Autodesk Inventor part; units mm, degrees
ref_plane "YZ Plane" through (0, 0, 0) normal (1, 0, 0) x (0, 1, 0)
ref_plane "XZ Plane" through (0, 0, 0) normal (0, 1, 0) x (-1, 0, 0)
ref_plane "XY Plane" through (0, 0, 0) normal (0, 0, 1) x (1, 0, 0)
sketch "Sketch1" plane through (0, 0, 0) normal (0, 0, 1) x (1, 0, 0)
  line L0 (0, 0) -> (0, 24.13)
  line L1 (0, 24.13) -> (24.13, 24.13)
  line L2 (24.13, 24.13) -> (24.13, 0)
  line L3 (24.13, 0) -> (0, 0)
  line L4 (0, 0) -> (0, 1.7526)
  line L5 (9.144, 1.7526) -> (14.986, 1.7526)
  line L6 (9.144, 1.7526) -> (9.271, 1.7526)
  line L7 (9.271, 1.7526) -> (14.859, 1.7526)
  line L8 (0, 0) -> (0, 7.62)
  line L9 (24.13, 0) -> (24.13, 7.62)
  line L10 (14.859, 7.62) -> (19.685, 7.62)
  line L11 (19.685, 7.62) -> (19.685, 12.319)
  line L12 (19.685, 12.319) -> (14.859, 12.319)
  line L13 (9.271, 7.62) -> (4.445, 7.62)
  line L14 (4.445, 7.62) -> (4.445, 12.319)
  line L15 (4.445, 12.319) -> (9.271, 12.319)
  line L16 (9.271, 7.62) -> (9.271, 1.7526)
  line L17 (14.859, 1.7526) -> (14.859, 7.62)
  line L18 (14.859, 12.319) -> (14.859, 15.748)
  line L19 (9.271, 12.319) -> (9.271, 15.748)
  line L20 (19.812, 15.748) -> (19.812, 19.685)
  line L21 (14.859, 15.748) -> (19.812, 15.748)
  line L22 (19.812, 19.685) -> (4.445, 19.685)
  line L23 (4.445, 19.685) -> (4.445, 15.748)
  line L24 (4.445, 15.748) -> (9.271, 15.748)
  dimension "d0" = 24.13
  dimension "d1" = 24.13
  dimension "d2" = 1.7526
  dimension "d3" = 9.144
  dimension "d5" = 0.127
  dimension "d6" = 5.588
  dimension "d7" = 7.62
  dimension "d8" = 7.62
  dimension "d9" = 4.826
  dimension "d10" = 4.699
  dimension "d11" = 4.826
  dimension "d12" = 4.699
  dimension "d13" = 5.8674
  dimension "d14" = 5.8674
  dimension "d15" = 3.429
  dimension "d16" = 3.429
  dimension "d18" = 3.937
sketch "Sketch2" plane through (0, 0, 0) normal (0, 0, 1) x (1, 0, 0)
  point P0 (0, 0)
extrude "Extrusion1" add sketch "Sketch1" along normal blind 152.4
chamfer "Chamfer1" distance 6.35 angle 45 4 edges at (0, 24.13, 76.2) (24.13, 24.13, 76.2) (24.13, 0, 76.2) (0, 0, 76.2)
sketch "Sketch3" plane through (6.35, 0, 0) normal (0, -1, 0) x (1, 0, 0)
  line L0 (17.78, 0) -> (17.78, 152.4)
  line L1 (17.78, 152.4) -> (17.78, 144.78)
  line L2 (17.78, 144.78) -> (-6.35, 144.78)
  line L3 (2.921, 0) -> (2.921, 152.4)
  line L4 (-6.35, 144.78) -> (-6.35, 137.16)
  line L5 (-6.35, 152.4) -> (-6.35, 0)
  line L6 (-6.35, 137.16) -> (17.78, 137.16)
  line L7 (17.78, 137.16) -> (17.78, 144.78)
  dimension "d24" = 7.62
  dimension "d25" = 7.62
extrude "Extrusion2" cut sketch "Sketch3" against normal blind 17.399
sketch "Sketch4" plane through (6.35, 0, 0) normal (0, -1, 0) x (1, 0, 0)
  line L0 (17.78, 144.78) -> (17.78, 137.16)
  line L1 (17.78, 137.16) -> (-6.35, 137.16)
  line L2 (-6.35, 137.16) -> (-6.35, 133.604)
  line L3 (-6.35, 133.604) -> (17.78, 133.604)
  line L4 (17.78, 133.604) -> (17.78, 137.16)
  point P0 (-6.35, 0)
  dimension "d28" = 3.556
extrude "Extrusion3" add sketch "Sketch4" against normal blind 1.7526
sketch "Sketch5" plane through (0, 6.35, 137.16) normal (-0.7071, -0.7071, 0) x (-0.7071, 0.7071, 0)
  point P0 (-4.4901, 137.16)
sketch "Sketch6" plane through (6.35, 0, 0) normal (0, -1, 0) x (1, 0, 0)
  point P0 (-6.35, 0)
sketch "Sketch7" plane through (6.35, 0, 0) normal (0, -1, 0) x (1, 0, 0)
  line L0 (17.78, 137.16) -> (13.1826, 137.16)
  line L1 (-6.35, 137.16) -> (-6.35, 0)
  line L2 (17.78, 137.16) -> (-6.35, 137.16)
  line L3 (-6.35, 137.16) -> (-6.35, 133.604)
  line L4 (-6.35, 133.604) -> (17.78, 133.604)
  line L5 (17.78, 133.604) -> (17.78, 137.16)
  dimension "d31" = 3.556
extrude "Extrusion4" add sketch "Sketch7" along normal blind 3.81
chamfer "Chamfer2" distance 2.54 angle 45 1 edges at (12.065, -3.81, 133.604)
sketch "Sketch8" plane through (24.13, 1.7526, 137.16) normal (1, 0, 0) x (0, 0, -1)
  point P0 (137.16, -1.7526)
sketch "Sketch9" plane through (6.35, 1.7526, 0) normal (0, 1, 0) x (1, 0, 0)
  line L0 (17.78, -137.16) -> (17.78, -133.604)
  line L1 (13.1826, -137.16) -> (17.78, -137.16)
  line L2 (17.78, -137.16) -> (13.1826, -137.16)
  line L3 (13.1826, -137.16) -> (13.1826, -133.604)
  line L4 (13.1826, -133.604) -> (17.78, -133.604)
  line L5 (17.78, -133.604) -> (17.78, -137.16)
  point P0 (-6.35, 0)
extrude "Extrusion5" add sketch "Sketch9" along normal blind 5.08
sketch "Sketch10" plane through (6.35, 1.7526, 0) normal (0, 1, 0) x (1, 0, 0)
  point P0 (-6.35, 0)
sketch "Sketch11" plane through (0, 1.7526, 133.604) normal (-1, 0, 0) x (0, 0, 1)
  point P0 (-133.604, -1.7526)
sketch "Sketch12" plane through (0, 1.7526, 133.604) normal (-1, 0, 0) x (0, 0, 1)
  point P0 (-133.604, -1.7526)
sketch "Sketch13" plane through (6.35, 1.7526, 0) normal (0, 1, 0) x (1, 0, 0)
  line L0 (-1.7526, -133.604) -> (-1.7526, -137.16)
  line L1 (-6.35, -133.604) -> (17.78, -133.604)
  line L2 (-1.7526, -137.16) -> (-1.7526, -133.604)
  line L3 (-1.7526, -133.604) -> (-6.35, -133.604)
  line L4 (-6.35, -133.604) -> (-6.35, -137.16)
  line L5 (-6.35, -137.16) -> (-1.7526, -137.16)
  point P0 (-6.35, 0)
extrude "Extrusion6" add sketch "Sketch13" along normal blind 5.08
properties part number "RIPnewslideholder"
Geometry check sheet. Reference: the model listing, model coordinates, mm. A direction names the side the tool comes from. Give positions to 0.01 mm unless a question says otherwise; leave off trailing zeros. Write each loop counter-clockwise with the first axis right and the second up, starting at its lowest first coordinate (ties: lowest second). Pieces come first, ordered by that corner, then holes.
1) Access from +Z, -Z, +X, -X, +Y, -Y to the whole of each face (thin tool, end or side, straight path). Record for faces 4 (the flat face through (22, 17.399, 141)), 5 (the flat face through (19.685, 10, 149)), 6 (the flat face through (3.22, 21, 75.13)).
2) Material ranges on L1, parallel to Y at x = 8.5, z = 24.5 (3 decimals); L2, parallel to Z at x = 9, y = 7.5; L3, parallel to X at y = 17.5, z = 89 (3 decimals), recorded low to high.
3) Release check for a two-part mould opening along Z. For faces 1 (the flat face through (2, 17.399, 141)), 2 (the flat face through (17, 15.748, 68)), 3 (the flat face through (9, 15, 0)) record: pulls with the +Z half, pulls with the -Z half, needs draft (parallel to the pull), parting line crosses it, or undercut.
4) Section check B-B, the plane x = 21.5. Record the boundary of the cut face in (y, z), and give its area (3 significant figures).
5) Section check A-A, the plane x = 11.5. Record the boundary of the cut face in (y, z) (3 decimals).
6) Gauge pin test, flat ends, axial feed: pin 1 (6 mm diameter, centred on y = 21.5, z = 46, fed in from +X); pin 2 (1 mm diameter, centred on y = 1.5, z = 119, fed in from -X); pin 3 (5 mm diameter, centred on x = 21, z = 130, fed in from +Y). Record the tip position at first contact, or that the pin passes through.
Computed:
1. face 4: +X, -X, -Y
1. face 5: +Z, -Z
1. face 6: +Z, -Z, -X, +Y
2. L1: y = 0 to 7.62, 12.319 to 15.748, 19.685 to 24.13
2. L2: z = 0 to 137.16, 144.78 to 152.4
2. L3: x = 0 to 4.445, 19.812 to 24.13
3. face 1: undercut
3. face 2: needs draft
3. face 3: pulls with the -Z half
4. outline: (-3.81, 136.14) - (-1.27, 133.6) - (3.72, 133.6) - (3.72, 0) - (20.41, 0) - (20.41, 152.4) - (3.72, 152.4) - (3.72, 144.78) - (17.4, 144.78) - (17.4, 137.16) - (-3.81, 137.16) - close
4. area: 2,460 mm2
5. outline: (-3.81, 136.144) - (-1.27, 133.604) - (0, 133.604) - (0, 0) - (1.753, 0) - (1.753, 137.16) - (-3.81, 137.16) - close; (0, 144.78) - (1.753, 144.78) - (1.753, 152.4) - (0, 152.4) - close; (19.685, 0) - (24.13, 0) - (24.13, 152.4) - (19.685, 152.4) - close
6. pin 1: stops at x = 23.41
6. pin 2: stops at x = 4.35
6. pin 3: stops at y = 23.41
